Work out the finished part from the listing and answer in its coordinate system (mm). A direction names the side the tool comes from. Round coordinates to 2 decimals unless told otherwise and drop trailing zeros. Order: outer loops, then holes, each group sorted by start corner. A loop starts at its lowest first (then second) coordinate and runs counter-clockwise, first axis right, second up. Notation, with made-up numbers: (-27, 23.25) - (-7, 23.25) arc R22 ccw to (-7, 39.25) - close; hole circle Ø2 at (-25, 5.5). An arc over 180 degrees is marked (long way). Answer in a Markdown table with one row per item.
from build123d import *

# Parameters (mm, degrees)
SKETCH1_W           = 35
SKETCH1_H           = 40
BOSS_EXTRUDE1_DEPTH = 2.9718
SKETCH2_W           = 5
SKETCH2_H           = 7
SKETCH2_W_2         = 10
SKETCH2_H_2         = 3.81
BOSS_EXTRUDE2_DEPTH = 2.9718
BOSS_EXTRUDE3_DEPTH = 2.9718
FILLET1_R           = 2
FILLET2_R           = 2
FILLET3_R           = 2
SKETCH4_W           = 3.302
SKETCH4_H           = 10
CUT_EXTRUDE1_DEPTH  = 3.9718


with BuildPart() as part:
    # Sketch1 → Boss-Extrude1 (new body)
    with BuildSketch(Plane.XY):
        Rectangle(SKETCH1_W, SKETCH1_H)
    extrude(amount=BOSS_EXTRUDE1_DEPTH)

    # Sketch2 → Boss-Extrude2 (add)
    with BuildSketch(Plane.XY.offset(2.9718)):
        Polygon((-3.900430119, 20), (7.099569881, 25), (9.099569881, 25), (9.099569881, 20), align=None)
        with Locations((-15, 23.5)):
            Rectangle(SKETCH2_W, SKETCH2_H)
        with Locations((-12.5, -21.905)):
            Rectangle(SKETCH2_W_2, SKETCH2_H_2)
        with Locations((12.5, -21.905)):
            Rectangle(SKETCH2_W_2, SKETCH2_H_2)
    extrude(amount=-BOSS_EXTRUDE2_DEPTH)

    # Sketch3 → Boss-Extrude3 (add)
    with BuildSketch(Plane.XY.offset(2.9718)):
        Polygon((-17.5, -20), (-27.5, -20), (-17.5, 1.595), align=None)
    extrude(amount=-BOSS_EXTRUDE3_DEPTH)

    # Fillet1
    fillet1_edges = [part.edges().sort_by_distance(p)[0] for p in [
        (-12.5, 20, 1.4859),
    ]]
    fillet(fillet1_edges, radius=FILLET1_R)

    # Fillet2
    fillet2_edges = [part.edges().sort_by_distance(p)[0] for p in [
        (9.099569881, 20, 1.4859),
    ]]
    fillet(fillet2_edges, radius=FILLET2_R)

    # Fillet3
    fillet3_edges = [part.edges().sort_by_distance(p)[0] for p in [
        (-17.5, 1.595, 1.4859),
    ]]
    fillet(fillet3_edges, radius=FILLET3_R)

    # Sketch4 → Cut-Extrude1 (cut, through all)
    with BuildSketch(Plane.XY.offset(2.9718)):
        with Locations((0, -15)):
            Rectangle(SKETCH4_W, SKETCH4_H)
    extrude(amount=-CUT_EXTRUDE1_DEPTH, mode=Mode.SUBTRACT)


solid = part.part
1) Find section A-A, the plane y = -13. Give the vertices of the cut face in (x, z).
Filled in:
| item | result |
|---|---|
| outline | (-24.26, 0) - (-1.65, 0) - (-1.65, 2.97) - (-24.26, 2.97) - close; (1.65, 0) - (17.5, 0) - (17.5, 2.97) - (1.65, 2.97) - close |
2) Each of these flat-tipped pins is pushed along its axis until it touches: pin 1 (1.5 mm diameter, centred on y = 25.5, z = 1.5, fed in from +X); pin 2 (1.5 mm diameter, centred on x = -20, z = 2, fed in from -Y); pin 3 (0.9 mm diameter, centred on y = -14.5, z = 1.5, fed in from -X). Where does it stop, or does it pass through?
Filled in:
| item | result |
|---|---|
| pin 1 | stops at x = 9.1 |
| pin 2 | stops at y = -20 |
| pin 3 | stops at x = -25.16 |
3) Find section B-B, the plane z = 0.6. Give the vertices of the cut face in (x, y), then the cut area to 3 significant figures.
Filled in:
| item | result |
|---|---|
| outline | (-27.5, -20) - (-17.5, -20) - (-17.5, -23.81) - (-7.5, -23.81) - (-7.5, -20) - (-1.65, -20) - (-1.65, -10) - (1.65, -10) - (1.65, -20) - (7.5, -20) - (7.5, -23.81) - (17.5, -23.81) - (17.5, 20) - (11.1, 20) arc R2 cw to (9.1, 22) - (9.1, 25) - (7.1, 25) - (-3.9, 20) - (-10.5, 20) arc R2 cw to (-12.5, 22) - (-12.5, 27) - (-17.5, 27) - (-17.5, 2.04) arc R2 cw to (-17.69, 1.2) - close |
| area | 1,630 mm^2 |
4) Which of the six approach directions +Z, -Z, +X, -X, +Y, -Y give full straight-line access (tool end or side, diameter ignored) to faces 5 (the face through (7.5, -22, 2)), 6 (the face through (-17.5, -22, 2)), 7 (the face through (1.523, 22.465, 1.507)), 8 (the face through (14, 20, 1))?
Filled in:
| item | result |
|---|---|
| face 5 | +Z, -Z, -Y |
| face 6 | +Z, -Z, -X, -Y |
| face 7 | +Z, -Z, +Y |
| face 8 | +Z, -Z, +X, +Y |
5) Find section D-D, the plane y = -19. Give the vertices of the cut face in (x, z).
Filled in:
| item | result |
|---|---|
| outline | (-27.04, 0) - (-1.65, 0) - (-1.65, 2.97) - (-27.04, 2.97) - close; (1.65, 0) - (17.5, 0) - (17.5, 2.97) - (1.65, 2.97) - close |
6) Find the intervals of material crossed by probe 1 along X at (y, z) = (14, 0.3); probe 2 along X at (y, z) = (-19, 2); probe 3 along X at (y, z) = (-16, 2.55), in increasing order. Write a range as from..to.
Filled in:
| item | result |
|---|---|
| probe 1 | x = -17.5..17.5 |
| probe 2 | x = -27.04..-1.65, 1.65..17.5 |
| probe 3 | x = -25.65..-1.65, 1.65..17.5 |
7) The mould has two halves that part along X. Classify faces 1 (the face through (1.651, -15, 2)), 2 (the face through (9.1, 24, 2)), 3 (the face through (-1.651, -15, 2)), 4 (the face through (-22.66, -9.55, 1.51)): released by +X, released by -X, zero draft, split by the parting line, or undercut.
Filled in:
| item | result |
|---|---|
| face 1 | undercut |
| face 2 | released by +X |
| face 3 | undercut |
| face 4 | released by -X |
8) Find section C-C, the plane x = -5. Give the vertices of the cut face in (y, z).
Filled in:
| item | result |
|---|---|
| outline | (-20, 0) - (20, 0) - (20, 2.97) - (-20, 2.97) - close |
